```python
from build123d import *

# Parameters (mm, degrees)
F1_DEPTH = 20
F2_R     = 62.5
F3_DEPTH = 4
F4_W     = 140
F4_H     = 4
F5_DEPTH = 12


# Not quite as in the source:
# - a feature of the source that left no trace in its solid (it failed there, or was rolled back) is left out


with BuildPart() as f1:
    # F0 (on Top) → F1 (new body)
    with BuildSketch(Plane.XY):
        with BuildLine():
            Line((80, -100), (80, 0))
            ThreePointArc((80, 0), (0, 80), (-80, 0))
            Line((-80, 0), (-80, -100))
            Line((-80, -100), (80, -100))
        make_face()
    extrude(amount=F1_DEPTH)

    # F2 (on face) → F3 (cut)
    with BuildSketch(Plane.XY.offset(20)):
        Circle(F2_R)
    extrude(amount=-F3_DEPTH, mode=Mode.SUBTRACT)

    # F4 (on face) → F5 (cut)
    with BuildSketch(Plane.XY.offset(20)):
        with Locations((0, -88)):
            Rectangle(F4_W, F4_H)
    extrude(amount=-F5_DEPTH, mode=Mode.SUBTRACT)


solid = f1.part
```
For this review, take the finished solid that the model builds, in its own axes (mm). A direction names the side the tool comes from. Give positions to 0.01 mm unless a question says otherwise; leave off trailing zeros. Write each loop counter-clockwise with the first axis right and the second up, starting at its lowest first coordinate (ties: lowest second). Pieces come first, ordered by that corner, then holes. Notation, with made-up numbers: M -15,39.25 L 37,39.25 A9 ccw 37,45.25 Z; hole C 9,-3 d9. An arc over 180 degrees is marked long. Answer as a JSON object with one key per item and string values. Group by question number.
Item 1: Consider section B-B on x = -15.5. Write out the cut boundary in (y, z).
Item 2: Draft analysis for pull direction Y (two halves, no side actions). For faces 1 (the flat face through (80, -51, 10)), 2 (the cylindrical face through (1.76, 79.98, 9.86)), 3 (the flat face through (-1, -90, 14)), state which applies: +Y half, -Y half, draft (parallel to the pull), parting line (faces both ways), or undercut.
Item 3: Consider section C-C on y = 53. Write out the cut boundary in (x, z).
Item 4: For pin 1 Ø3.5 at (x, z) = (12, 15) entering from +Y; pin 2 Ø4 at (y, z) = (20.5, 17) entering from -X; pin 3 Ø5 at (x, z) = (30.5, 14.5) entering from +Y, all flat-tipped, find the tip position at first contact; note any pin that passes through.
Item 5: Consider section D-D on x = 67. Write out the cut boundary in (y, z), plus the area to 3 significant figures.
Item 6: For probe 1 along Y at (x, z) = (0, 18.95); probe 2 along Y at (x, z) = (33.5, 17); probe 3 along Z at (x, y) = (60, -16), list the stretches that pass through material, from the lowest coordinate up. Write a range as [from, to].
Item 7: Tool access review of faces 4 (the cylindrical face through (-62.44, 2.75, 18.03)), 5 (the flat face through (-1, -69, 20)): name each direction out of +Z, -Z, +X, -X, +Y, -Y from which nothing blocks a thin tool from reaching the whole face with its end or side.
Item 8: Consider section A-A on z = 10.25. Write out the cut boundary in (x, y), plus the area to 3 significant figures.
Check result:
{
 "1": {"outline": "M -100,0 L 78.48,0 L 78.48,20 L 60.55,20 L 60.55,16 L -60.55,16 L -60.55,20 L -86,20 L -86,8 L -90,8 L -90,20 L -100,20 Z"},
 "2": {"face 1": "draft", "face 2": "+Y half", "face 3": "undercut"},
 "3": {"outline": "M -59.92,0 L 59.92,0 L 59.92,20 L 33.12,20 L 33.12,16 L -33.12,16 L -33.12,20 L -59.92,20 Z"},
 "4": {"pin 1": "stops at y = 79.34", "pin 2": "stops at x = -77.83", "pin 3": "stops at y = 74.94"},
 "5": {"outline": "M -100,0 L 43.71,0 L 43.71,20 L -86,20 L -86,8 L -90,8 L -90,20 L -100,20 Z", "area": "2,830 mm^2"},
 "6": {"probe 1": "y = [-100, -90], [-86, -62.5], [62.5, 80]", "probe 2": "y = [-100, -90], [-86, -52.76], [52.76, 72.65]", "probe 3": "z = [0, 16]"},
 "7": {"face 4": "+Z", "face 5": "+Z, +X, -X, +Y, -Y"},
 "8": {"outline": "M -80,-100 L 80,-100 L 80,0 A80 ccw -80,0 Z; hole M -70,-90 L 70,-90 L 70,-86 L -70,-86 Z", "area": "25,500 mm^2"}
}
